from build123d import *

# Parameters (mm, degrees)
BOSS_EXTRUDE1_DEPTH = 3.175
SKETCH2_W           = 3.302
SKETCH2_H           = 33.02
SKETCH2_R           = 1.778
CUT_EXTRUDE1_DEPTH  = 195.021684248
SKETCH3_R           = 1.524
CUT_EXTRUDE2_DEPTH  = 195.021684248
SKETCH4_R           = 1.143
CUT_EXTRUDE3_DEPTH  = 195.021684248
FILLET1_R           = 12.7
SKETCH5_W           = 12.7
SKETCH5_H           = 3.175
CUT_EXTRUDE4_DEPTH  = 179.341965104
CUT_EXTRUDE5_DEPTH  = 179.341965104
SKETCH9_W           = 7.62
SKETCH9_H           = 15
CUT_EXTRUDE8_DEPTH  = 179.341965104


with BuildPart() as part:
    # Sketch1 → Boss-Extrude1 (new body)
    with BuildSketch(Plane(origin=(0, 0, 0), x_dir=(1, 0, 0), z_dir=(0, 1, 0))):
        Polygon((0, 146.646968374), (-127, -73.323484187), (127, -73.323484187), align=None)
    extrude(amount=BOSS_EXTRUDE1_DEPTH)

    # Sketch2 → Cut-Extrude1 (cut, through all)
    with BuildSketch(Plane(origin=(0, 3.175, 0), x_dir=(1, 0, 0), z_dir=(0, 1, 0))):
        with Locations((-17.907, 36.399572365)):
            Rectangle(SKETCH2_W, SKETCH2_H)
        with Locations(Location((-45.522797213, 43.314369578, 0), (0, 0, 270))):
            Circle(SKETCH2_R)
        with Locations(Location((-45.522797213, 29.484775151, 0), (0, 0, 270))):
            Circle(SKETCH2_R)
        with Locations(Location((-14.749945797, -61.081083627, 0), (0, 0, 270))):
            Circle(SKETCH2_R)
        with Locations(Location((-2.773165699, -54.166286414, 0), (0, 0, 270))):
            Circle(SKETCH2_R)
        Polygon((-7.445874938, -26.882511029), (-9.096874938, -24.022895146), (-37.693033771, -40.532895146), (-36.042033771, -43.392511029), align=None)
        Polygon((55.600033771, -9.517061335), (27.003874938, 6.992938665), (25.352874938, 4.133322782), (53.949033771, -12.376677218), align=None)
        with Locations(Location((48.295962913, 24.681511262, 0), (0, 0, 270))):
            Circle(SKETCH2_R)
        with Locations(Location((60.27274301, 17.766714049, 0), (0, 0, 270))):
            Circle(SKETCH2_R)
    extrude(amount=-CUT_EXTRUDE1_DEPTH, mode=Mode.SUBTRACT)

    # Sketch3 → Cut-Extrude2 (cut, through all)
    with BuildSketch(Plane(origin=(0, 3.175, 0), x_dir=(1, 0, 0), z_dir=(0, 1, 0))):
        with Locations(Location((0, 118.312139176, 0), (0, 0, 270))):
            Circle(SKETCH3_R)
        with Locations(Location((-102.461318102, -59.156069588, 0), (0, 0, 270))):
            Circle(SKETCH3_R)
        with Locations(Location((102.461318102, -59.156069588, 0), (0, 0, 270))):
            Circle(SKETCH3_R)
    extrude(amount=-CUT_EXTRUDE2_DEPTH, mode=Mode.SUBTRACT)

    # Sketch4 → Cut-Extrude3 (cut, through all)
    with BuildSketch(Plane(origin=(0, 3.175, 0), x_dir=(1, 0, 0), z_dir=(0, 1, 0))):
        with Locations(Location((0, 8.207705491, 0), (0, 0, 270))):
            Circle(SKETCH4_R)
        with Locations(Location((16.51, -6.397294509, 0), (0, 0, 270))):
            Circle(SKETCH4_R)
    extrude(amount=-CUT_EXTRUDE3_DEPTH, mode=Mode.SUBTRACT)

    # Fillet1
    fillet1_edges = [part.edges().sort_by_distance(p)[0] for p in [
        (127, 1.5875, 73.323484187),
        (-127, 1.5875, 73.323484187),
        (0, 1.5875, -146.646968374),
    ]]
    fillet(fillet1_edges, radius=FILLET1_R)

    # Sketch5 → Cut-Extrude4 (cut, through all)
    with BuildSketch(Plane(origin=(0, 3.175, 0), x_dir=(1, 0, 0), z_dir=(0, 1, 0))):
        with Locations((-57.15, -69.195984187)):
            Rectangle(SKETCH5_W, SKETCH5_H)
        with Locations((57.15, -69.195984187)):
            Rectangle(SKETCH5_W, SKETCH5_H)
        Polygon((92.931850743, -19.395718754), (86.581850743, -8.397196126), (83.832220086, -9.984696126), (90.182220086, -20.983218754), align=None)
        Polygon((33.032220086, 78.003484899), (35.781850743, 79.590984899), (29.431850743, 90.589507527), (26.682220086, 89.002007527), align=None)
        Polygon((-29.550295474, 90.384355234), (-35.900295474, 79.385832606), (-33.150664817, 77.798332606), (-26.800664817, 88.796855234), align=None)
        Polygon((-83.950664817, -10.189848419), (-86.700295474, -8.602348419), (-93.050295474, -19.600871047), (-90.300664817, -21.188371047), align=None)
    extrude(amount=-CUT_EXTRUDE4_DEPTH, mode=Mode.SUBTRACT)

    # Sketch6 → Cut-Extrude5 (cut, through all)
    with BuildSketch(Plane(origin=(0, 3.175, 0), x_dir=(1, 0, 0), z_dir=(0, 1, 0))):
        Polygon((-54.829873821, -11.096773597), (-45.329873821, 5.357709075), (-56.988307807, 12.088709075), (-66.488307807, -4.365773597), align=None)
    extrude(amount=-CUT_EXTRUDE5_DEPTH, mode=Mode.SUBTRACT)

    # Sketch9 → Cut-Extrude8 (cut, through all)
    with BuildSketch(Plane(origin=(0, 3.175, 0), x_dir=(1, 0, 0), z_dir=(0, 1, 0))):
        with Locations((6.254067487, 57.836284876)):
            Rectangle(SKETCH9_W, SKETCH9_H)
    extrude(amount=-CUT_EXTRUDE8_DEPTH, mode=Mode.SUBTRACT)


solid = part.part
Source: CAD feature listing. Evaluate the final solid. Frame: model axes, mm. A direction names the side the tool comes from. Coordinates: 2 decimals unless noted, no trailing zeros. Loops run counter-clockwise (first coordinate to the right, second up) from the corner with the lowest first, then second, coordinate; pieces in that order, holes last. Notation, with made-up numbers: (24.25, -4.75) - (44.25, -4.75) arc R15 ccw to (44.25, 19.25) - close; hole circle Ø10 at (12, -10.5). An arc over 180 degrees is marked (long way). One line per item, written item: value. Start each with the question number.
1. Section D-D (x = -71). Return the cut outline in (y, z) (3 decimals), and give its area (3 significant figures).
2. Section C-C (z = 31). Return the cut outline in (x, y) (3 decimals), and give its area (3 significant figures).
3. Section A-A (z = -56). Return the cut outline in (x, y) (3 decimals), and give its area (3 significant figures).
4. Contact query for flat-ended pins moving along their axis: P1, Ø10, axis at x = -56, z = -57, coming from the +Y side (3 decimals); P2, Ø1, axis at y = 2.5, z = -35.5, coming from the -X side; P3, Ø1, axis at x = 87.5, y = 0.5, coming from the -Z side; P4, Ø1.6, axis at y = 1.5, z = 68.5, coming from the -X side. Output: stop coordinate, or through.
5. Mould query, pull axis Z, two halves, no side actions, for faces 3 (the flat face through (-62.765, 1.565, -37.935)), 4 (the flat face through (-87.17, 1.61, 15.766)), 5 (the cylindrical face through (-116.1, 1.6, 66.8)). Classes: pulls with the +Z half, pulls with the -Z half, needs draft (parallel to the pull), parting line crosses it, or undercut.
6. Section B-B (y = 1.2). State how many separate pieces and enclosed holes the cut face has, and give its area (3 significant figures).
7. Set-up query: faces 1 (the flat face through (-21.94, 1.61, 35.25)), 2 (the flat face through (64.235, 1.565, -35.389)). Return all of +Z, -Z, +X, -X, +Y, -Y with unobstructed straight access to the full face (end or side cutting, diameter ignored); none if empty.
8. Ray query, L1, parallel to Z at x = 28, y = 1.1 (3 decimals); L2, parallel to X at y = 0.95, z = -24.5; L3, parallel to X at y = 1.3, z = -88.5. Return the intervals inside material, ascending.
Verdict:
1. outline: (0, -23.671) - (3.175, -23.671) - (3.175, 73.323) - (0, 73.323) - close
1. area: 308 mm2
2. outline: (-102.565, 0) - (-21.182, 0) - (-21.182, 3.175) - (-102.565, 3.175) - close; (-14.578, 0) - (102.565, 0) - (102.565, 3.175) - (-14.578, 3.175) - close
2. area: 630 mm2
3. outline: (-52.335, 0) - (2.444, 0) - (2.444, 3.175) - (-52.335, 3.175) - close; (10.064, 0) - (52.335, 0) - (52.335, 3.175) - (10.064, 3.175) - close
3. area: 308 mm2
4. P1: stops at y = 3.175
4. P2: stops at x = -64.46
4. P3: stops at z = 4.04
4. P4: stops at x = -115.55
5. face 3: pulls with the -Z half
5. face 4: undercut
5. face 5: parting line crosses it
6. separate pieces: 1
6. enclosed holes: 22
6. area: 26,600 mm2
7. face 1: +Y, -Y
7. face 2: -Z, +X, +Y, -Y
8. L1: z = -98.15 to -89.763, -86.72 to -6.418, -2.605 to 73.323
8. L2: x = -70.52 to -19.56, -16.26 to 46.53, 50.06 to 70.52
8. L3: x = -33.57 to -30.64, -26.97 to 26.97, 30.64 to 33.57
